Geometry check sheet. Reference: drawing and pictorial views, mm from the part's lowest x, y, z. Round coordinates to 2 decimals unless told otherwise and drop trailing zeros. Write each loop counter-clockwise with the first axis right and the second up, starting at its lowest first coordinate (ties: lowest second). Pieces come first, ordered by that corner, then holes. Notation, with made-up numbers: (51.5, 26.25) -> (80.5, 26.25) arc R4 cw to (80.5, 31.25) -> close; hole circle Ø6 at (7, 81.5). An arc over 180 degrees is marked (long way). Answer as a JSON object with one key per item and string values. Group by question number.
(1) Scan lines: L1, parallel to X at y = 50.8, z = 125 (1 decimal); L2, parallel to Z at x = 11, y = 66.5; L3, parallel to Y at x = 50, z = 102. Record each from-to range of solid material in increasing order. Write a range as from..to.
(2) Sectioned sample at D-D on y = 92. Record the cut outline in (x, z).
(3) Gauge pin test, flat ends, axial feed: pin 1 Ø8 at (y, z) = (32.5, 100.5) entering from -X; pin 2 Ø4 at (y, z) = (69, 85.5) entering from -X; pin 3 Ø5 at (x, y) = (77, 79.5) entering from +Z. Record the tip position at first contact, or that the pin passes through.
(4) Sectioned sample at B-B on x = 65.5. Record the cut outline in (y, z).
(5) Draft check along X on the marked faces 1, 2 and 3. Enter one of: released by +X, released by -X, zero draft, split by the parting line, or undercut.
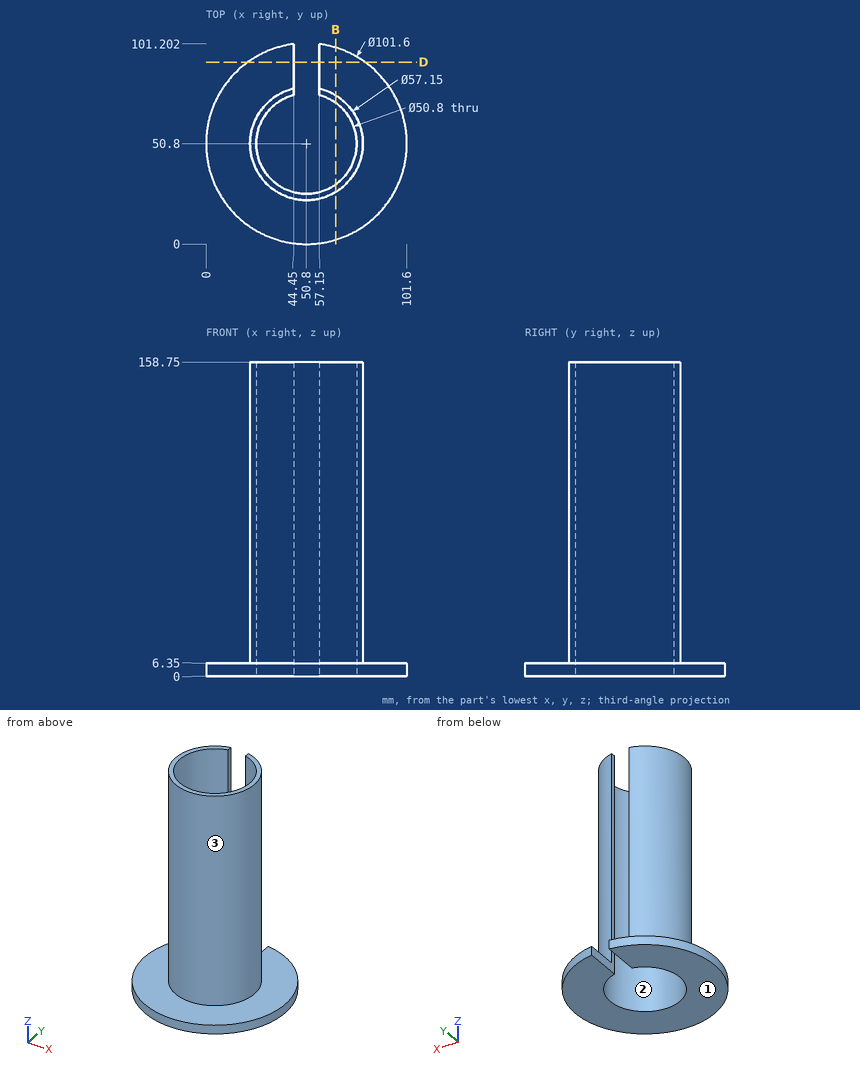
Computed values:
{
 "1": {"L1": "22.2..25.4, 76.2..79.4", "L2": "0..6.35", "L3": "22.24..25.41"},
 "2": {"outline": "(21.08, 0) -> (44.45, 0) -> (44.45, 6.35) -> (21.08, 6.35) -> close; (57.15, 0) -> (80.52, 0) -> (80.52, 6.35) -> (57.15, 6.35) -> close"},
 "3": {"pin 1": "x = 26.06", "pin 2": "x = 27.26", "pin 3": "z = 6.35"},
 "4": {"outline": "(2.17, 0) -> (30.09, 0) -> (30.09, 158.75) -> (26.3, 158.75) -> (26.3, 6.35) -> (2.17, 6.35) -> close; (71.51, 0) -> (99.43, 0) -> (99.43, 6.35) -> (75.3, 6.35) -> (75.3, 158.75) -> (71.51, 158.75) -> close"},
 "5": {"face 1": "zero draft", "face 2": "undercut", "face 3": "split by the parting line"}
}
